Input: part model. Units: mm. Frame: model coordinates. Face numbers are marked on the shaded views. A direction names the side the tool comes from. Coordinates: 2 decimals unless noted, no trailing zeros. Write each loop counter-clockwise with the first axis right and the second up, starting at its lowest first coordinate (ties: lowest second). Pieces come first, ordered by that corner, then holes.
1) Section query B-B (y = 0). Output: boundary loops of the cut face in (x, z), then the cut area to 3 significant figures.
2) Set-up query: the marked faces 1 and 2. Return all of +Z, -Z, +X, -X, +Y, -Y with unobstructed straight access to the full face (end or side cutting, diameter ignored); none if empty.
3) Section query D-D (x = 6.5). Output: boundary loops of the cut face in (y, z), then the cut area to 3 significant figures.
4) Pin query (flat end, axial travel): pin 1 Ø1 at (x, z) = (5, -0.5) entering from -Y; pin 2 Ø5 at (x, y) = (0, 0) entering from +Z; pin 3 Ø1 at (x, z) = (5.5, -1.5) entering from -Y; pin 4 Ø1.5 at (y, z) = (5, 4) entering from -X. Return the tip coordinate at first contact, or that it passes through.
5) Section query C-C (z = -1.25). Output: boundary loops of the cut face in (x, y).
6) Draft query along X for the marked faces 3 and 4. Return one class per face: pulls with the +X half, pulls with the -X half, needs draft (parallel to the pull), parting line crosses it, or undercut.
7) Line query: L1, parallel to X at y = -1.75, z = 5.75; L2, parallel to Z at x = -1.25, y = -6; L3, parallel to Y at x = -1.5, z = 3.5. Output: solid intervals per line, ascending.
8) Section query A-A (x = 0). Output: boundary loops of the cut face in (y, z).
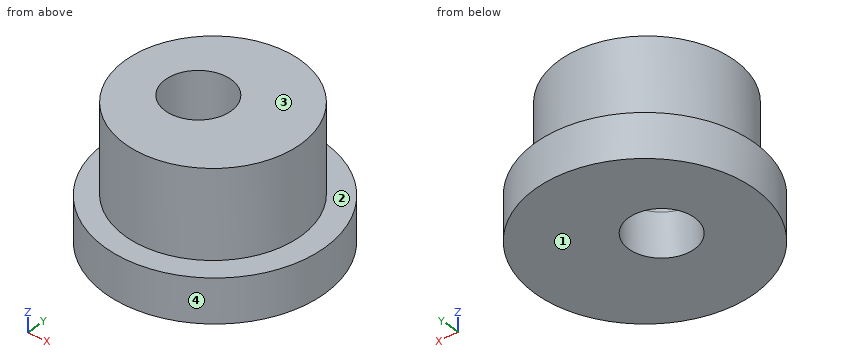
from build123d import *

# Parameters (mm, degrees)
F0_R     = 6
F0_R_2   = 2.25
F1_DEPTH = 6
F2_R     = 7.5
F2_R_2   = 6
F3_DEPTH = 3


with BuildPart() as f1:
    # F0 (on Top) → F1 (new body)
    with BuildSketch(Plane.XY):
        with Locations((1, 0)):
            Circle(F0_R)
        Circle(F0_R_2, mode=Mode.SUBTRACT)
    extrude(amount=F1_DEPTH)

    # F2 (on face) + F0 (on Top) → F3 (join)
    with BuildSketch(Plane.XY):
        with Locations((1.137572, 0)):
            Circle(F2_R)
        with Locations((1, 0)):
            Circle(F2_R_2, mode=Mode.SUBTRACT)
    with BuildSketch(Plane.XY):
        with Locations((1, 0)):
            Circle(F0_R)
        Circle(F0_R_2, mode=Mode.SUBTRACT)
    extrude(amount=-F3_DEPTH)


solid = f1.part
Answer:
1. outline: (-6.36, -3) - (-2.25, -3) - (-2.25, 6) - (-5, 6) - (-5, 0) - (-6.36, 0) - close; (2.25, -3) - (8.64, -3) - (8.64, 0) - (7, 0) - (7, 6) - (2.25, 6) - close
1. area: 76.5 mm2
2. face 1: -Z, +X, -X, +Y, -Y
2. face 2: +Z
3. outline: (-5.24, -3) - (5.24, -3) - (5.24, 0) - (2.4, 0) - (2.4, 6) - (-2.4, 6) - (-2.4, 0) - (-5.24, 0) - close
3. area: 60.2 mm2
4. pin 1: stops at y = -6.7
4. pin 2: stops at z = 6
4. pin 3: stops at y = -6.43
4. pin 4: stops at x = -3.24
5. outline: circle Ø15 at (1.14, 0); hole circle Ø4.5 at (0, 0)
6. face 3: needs draft
6. face 4: parting line crosses it
7. L1: x = -4.74 to -1.41, 1.41 to 6.74
7. L2: z = -3 to 0
7. L3: y = -5.45 to -1.68, 1.68 to 5.45
8. outline: (-7.41, -3) - (-2.25, -3) - (-2.25, 6) - (-5.92, 6) - (-5.92, 0) - (-7.41, 0) - close; (2.25, -3) - (7.41, -3) - (7.41, 0) - (5.92, 0) - (5.92, 6) - (2.25, 6) - close
